Source: CAD feature listing. Evaluate the final solid. Frame: model axes, mm. Coordinates: 2 decimals unless noted, no trailing zeros. Loops run counter-clockwise (first coordinate to the right, second up) from the corner with the lowest first, then second, coordinate; pieces in that order, holes last. Notation, with made-up numbers: M 82,2 L 104,2 A16 ccw 104,10 Z; hole C -13.5,5.5 d11. An arc over 180 degrees is marked long. Write each question's results on one line, items separated by ' | '. Start each with the question number.
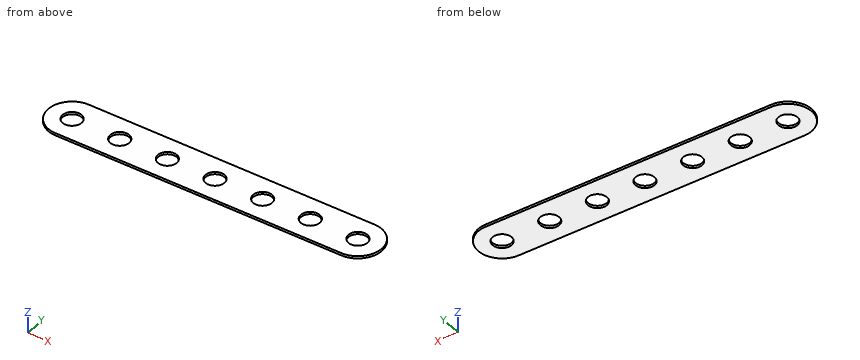
Autodesk Inventor part; units mm, degrees
ref_plane "YZ Plane" through (0, 0, 0) normal (1, 0, 0) x (0, 1, 0)
ref_plane "XZ Plane" through (0, 0, 0) normal (0, 1, 0) x (-1, 0, 0)
ref_plane "XY Plane" through (0, 0, 0) normal (0, 0, 1) x (1, 0, 0)
sketch "Náčrt1" plane through (0, 0, 0) normal (0, 0, 1) x (1, 0, 0)
  line L0 (-30, 0) -> (30, 0) construction
  line L1 (-30, -5) -> (30, -5)
  line L2 (30, 5) -> (-30, 5)
  arc A0 (-30, 5) -> (-30, -5) centre (-30, 0) ccw
  arc A1 (30, -5) -> (30, 5) centre (30, 0) ccw
  point P0 (0, 0)
  point P1 (35, 0)
  dimension "d0" = 35
  dimension "d1" = 5
extrude "Vysunutí1" add sketch "Náčrt1" along normal blind 0.5
sketch "Náčrt2" plane through (0, 0, 0) normal (0, 0, -1) x (-1, 0, 0)
  arc A0 (30, -5) -> (30, 5) centre (30, 0) ccw
  circle A1 centre (30, 0) radius 2
  point P0 (0, 0)
  dimension "d4" = 4
extrude "Vysunutí2" cut sketch "Náčrt2" against normal through all
pattern_linear "Obdélníkové pole1" count 7 spacing 10 along (1, 0, 0) of "Vysunutí2"
properties part number "1007"
Item 1: Cut plane C-C (x = -9). Output: boundary loops of the cut face in (y, z).
Item 2: Line query: probe 1 along Y at (x, z) = (20, 0.1); probe 2 along Y at (x, z) = (-8.5, 0.4); probe 3 along X at (y, z) = (-3.25, 0.3). Output: solid intervals per line, ascending.
Item 3: Cut plane D-D (y = 3.25). Output: boundary loops of the cut face in (x, z), then the cut area to 3 significant figures.
Item 4: Cut plane B-B (z = 0.3). Output: boundary loops of the cut face in (x, y), then the cut area to 3 significant figures.
Item 5: Cut plane A-A (x = -20). Output: boundary loops of the cut face in (y, z).
Response values:
1) outline: M -5,0 L -1.73,0 L -1.73,0.5 L -5,0.5 Z; M 1.73,0 L 5,0 L 5,0.5 L 1.73,0.5 Z
2) probe 1: y = -5 to -2, 2 to 5 | probe 2: y = -5 to -1.32, 1.32 to 5 | probe 3: x = -33.8 to 33.8
3) outline: M -33.8,0 L 33.8,0 L 33.8,0.5 L -33.8,0.5 Z | area: 33.8 mm2
4) outline: M -30,-5 L 30,-5 A5 ccw 30,5 L -30,5 A5 ccw Z; hole C -30,0 d4; hole C -20,0 d4; hole C -10,0 d4; hole C 0,0 d4; hole C 10,0 d4; hole C 20,0 d4; hole C 30,0 d4 | area: 591 mm2
5) outline: M -5,0 L -2,0 L -2,0.5 L -5,0.5 Z; M 2,0 L 5,0 L 5,0.5 L 2,0.5 Z
